from build123d import *

# Parameters (mm, degrees)
F3_DEPTH = 6.351


with BuildPart() as f1:
    # F0 (on Top) → F1 (revolve)
    with BuildSketch(Plane.XY):
        with BuildLine():
            Line((7.62, 0), (6.35, 0))
            Line((6.35, 0), (6.35, 1.524))
            Line((6.35, 1.524), (7.14375, 3.226202))
            Line((7.14375, 3.226202), (6.35, 6.35))
            ThreePointArc((6.35, 6.35), (5.451974, 5.978026), (5.08, 5.08))
            Line((5.08, 5.08), (5.08, 0))
            ThreePointArc((5.08, 0), (6.35, -1.27), (7.62, 0))
        make_face()
    revolve(axis=Axis((0, 3.175, 0), (0, 1, 0)))

    # F2 (on Front) → F3 (cut, through all)
    with BuildSketch(Plane.XZ):
        Polygon((-1.374815, 0.79375), (-0.458272, 0.79375), (0, 1.5875), (-5.662592, 11.395398), (-7.037408, 10.601648), align=None)
        Polygon((0, 1.5875), (0.458272, 0.79375), (1.374815, 0.79375), (7.037408, 10.601648), (5.662592, 11.395398), align=None)
        Polygon((-0.916544, 0), (-1.374815, 0.79375), (-12.7, 0.79375), (-12.7, -0.79375), (-1.374815, -0.79375), align=None)
        Polygon((12.7, 0.79375), (1.374815, 0.79375), (0.916544, 0), (1.374815, -0.79375), (12.7, -0.79375), align=None)
        Polygon((0, -1.5875), (-0.458272, -0.79375), (-1.374815, -0.79375), (-7.037408, -10.601648), (-5.662592, -11.395398), align=None)
        Polygon((1.374815, -0.79375), (0.458272, -0.79375), (0, -1.5875), (5.662592, -11.395398), (7.037408, -10.601648), align=None)
    extrude(amount=-F3_DEPTH, mode=Mode.SUBTRACT)


solid = f1.part
Read the model definition and answer for the solid it produces. Units are mm, in the model's axes. A direction names the side the tool comes from. Round coordinates to 2 decimals unless told otherwise and drop trailing zeros. Write each loop counter-clockwise with the first axis right and the second up, starting at its lowest first coordinate (ties: lowest second). Pieces come first, ordered by that corner, then holes.
1. The part is cut by section A-A, the plane x = 0. Determine the outline of the cut face in (y, z).
2. The part is cut by section C-C, the plane y = 5.75. Determine the outline of the cut face in (x, z), then the cut area to 3 significant figures.
3. The part is cut by section D-D, the plane z = 5.5. State how many separate pieces and enclosed holes the cut face has, then the cut area to 3 significant figures.
4. Given pin 1 Ø2.5 at (x, y) = (6, 3) entering from -Z; pin 2 Ø1 at (x, y) = (-1.5, 2.5) entering from +Z; pin 3 Ø4 at (x, z) = (6, 4.5) entering from +Y; pin 4 Ø3 at (y, z) = (5, 5.5) entering from -X, each flat-ended and moving along its own axis, determine where each tip first touches the part or whether it passes through.
5. Straight lines are drawn through the part: L1, parallel to Z at x = -1, y = 3.5; L2, parallel to Z at x = -3.75, y = 4; L3, parallel to X at y = 1, z = 2.5. For each, find the intervals that lie inside material, in ascending order.
6. Which of the six approach directions +Z, -Z, +X, -X, +Y, -Y give full straight-line access (tool end or side, diameter ignored) to faces 4 (the face through (4.41, 2.5, -2.52)), 5 (the face through (6, 3, 0.794)), 6 (the face through (5.9, 2.4, -3.3))?
7. Determine the mould class of faces 1 (the face through (3.594, 3.131, 4.637)), 2 (the face through (-5.858, 4.81, 3.337)), 3 (the face through (-0.039, 2.387, 6.752)) for opening direction Y: pulls with the +Y half, pulls with the -Y half, needs draft (parallel to the pull), parting line crosses it, or undercut.
8. The part is cut by section B-B, the plane y = 2.75. Determine the outline of the cut face in (x, z).
Values:
1. outline: (0, -7.62) - (0, -6.35) - (1.52, -6.35) - (3.23, -7.14) - (6.35, -6.35) arc R1.27 ccw to (5.08, -5.08) - (0, -5.08) arc R1.27 ccw to start; (0, 5.08) - (5.08, 5.08) arc R1.27 ccw to (6.35, 6.35) - (3.23, 7.14) - (1.52, 6.35) - (0, 6.35) - (0, 7.62) arc R1.27 ccw to start
2. outline: (-6.45, -0.79) arc R6.5 ccw to (-3.91, -5.19) - (-3.29, -4.12) arc R5.27 cw to (-5.21, -0.79) - close; (-6.45, 0.79) - (-5.21, 0.79) arc R5.27 cw to (-3.29, 4.12) - (-3.91, 5.19) arc R6.5 ccw to start; (-2.54, -5.99) arc R6.5 ccw to (2.54, -5.99) - (1.92, -4.91) arc R5.27 cw to (-1.92, -4.91) - close; (-2.54, 5.99) - (-1.92, 4.91) arc R5.27 cw to (1.92, 4.91) - (2.54, 5.99) arc R6.5 ccw to start; (3.29, -4.12) - (3.91, -5.19) arc R6.5 ccw to (6.45, -0.79) - (5.21, -0.79) arc R5.27 cw to start; (3.29, 4.12) arc R5.27 cw to (5.21, 0.79) - (6.45, 0.79) arc R6.5 ccw to (3.91, 5.19) - close
2. area: 33.8 mm2
3. separate pieces: 3
3. enclosed holes: 0
3. area: 39.8 mm2
4. pin 1: stops at z = -5.32
4. pin 2: stops at z = 6.9
4. pin 3: stops at y = 6.35
4. pin 4: stops at x = -5.46
5. L1: z = -7 to -4.98, 4.98 to 7
5. L2: z = -4.91 to -3.43, 3.43 to 4.91
5. L3: x = -5.84 to -4.42, 4.42 to 5.84
6. face 4: +Y, -Y
6. face 5: +X, -X, +Y
6. face 6: -Z, +X
7. face 1: needs draft
7. face 2: pulls with the +Y half
7. face 3: undercut
8. outline: (-6.88, -0.79) arc R6.92 ccw to (-4.13, -5.56) - (-3.2, -3.95) arc R5.08 cw to (-5.02, -0.79) - close; (-6.88, 0.79) - (-5.02, 0.79) arc R5.08 cw to (-3.2, 3.95) - (-4.13, 5.56) arc R6.92 ccw to start; (-2.75, -6.35) arc R6.92 ccw to (2.75, -6.35) - (1.82, -4.74) arc R5.08 cw to (-1.82, -4.74) - close; (-2.75, 6.35) - (-1.82, 4.74) arc R5.08 cw to (1.82, 4.74) - (2.75, 6.35) arc R6.92 ccw to start; (3.2, -3.95) - (4.13, -5.56) arc R6.92 ccw to (6.88, -0.79) - (5.02, -0.79) arc R5.08 cw to start; (3.2, 3.95) arc R5.08 cw to (5.02, 0.79) - (6.88, 0.79) arc R6.92 ccw to (4.13, 5.56) - close
